Read the model definition and answer for the solid it produces. Units are mm, in the model's axes. A direction names the side the tool comes from. Give positions to 0.01 mm unless a question says otherwise; leave off trailing zeros. Loops run counter-clockwise (first coordinate to the right, second up) from the corner with the lowest first, then second, coordinate; pieces in that order, holes last. Notation, with made-up numbers: (7.25, 51) - (56.25, 51) arc R25 cw to (56.25, 72) - close; hole circle Ø4 at (3.25, -6.5). An arc over 180 degrees is marked (long way). Use a Markdown table: item, result. Add a question column.
Item 1: Which of the six approach directions +Z, -Z, +X, -X, +Y, -Y give full straight-line access (tool end or side, diameter ignored) to faces 4 (the face through (-12.97, -1.89, -1.45)), 5 (the face through (0.13, 4.08, 1.88)), 6 (the face through (13.07, -1.89, -1.45))?
Item 2: A cutting plane is placed at B-B (x = 2). Determine the outline of the cut face in (y, z) (3 decimals).
Item 3: A cutting plane is placed at C-C (z = 0). Determine the outline of the cut face in (x, y) (3 decimals), plus the area to 3 significant figures.
Item 4: Consider probe 1 along Z at (x, y) = (5.75, 0) (3 decimals); probe 2 along Z at (x, y) = (-8.5, 4.5); probe 3 along Y at (x, z) = (-8, -5). Determine where each line is inside the solid, lowest interval first. Write a range as [from, to].
Item 5: For a pull along Z with two mould halves and no side action, classify faces 1 (the face through (0.112, -2.808, -12.646)), 2 (the face through (16.51, 0, 0)), 3 (the face through (0.13, -3.67, -5.03)) as +Z half, -Z half, draft (parallel to the pull), parting line (faces both ways), or undercut.
Item 6: A cutting plane is placed at D-D (z = -3.81). Give the number of separate pieces and of enclosed holes in the cut face, plus the area to 3 significant figures.
Item 7: Each of these flat-tipped pins is pushed along its axis until it touches: P1, Ø4, axis at y = 6.6, z = 3.81, coming from the -X side; P2, Ø4, axis at x = -3, z = 10.5, coming from the -Y side; P3, Ø8.5, axis at y = -6.6, z = -3.81, coming from the -X side (3 decimals); P4, Ø5, axis at x = 5, z = -8.5, coming from the -Y side. Where does it stop, or does it pass through?
Item 8: A cutting plane is placed at A-A (y = 0). Determine the outline of the cut face in (x, z) (3 decimals), plus the area to 4 significant figures.
from build123d import *

# Parameters (mm, degrees)
F0_R     = 12.954
F0_R_2   = 2.38125
F1_DEPTH = 9.525
F2_DEPTH = 16.51
F3_R     = 3.175
F4_DEPTH = 26.036
F5_SIZE  = 1.524


with BuildPart() as f1:
    # F0 (on Right) → F1 (new body, symmetric)
    with BuildSketch(Plane.YZ):
        Circle(F0_R)
        Circle(F0_R_2, mode=Mode.SUBTRACT)
    extrude(amount=F1_DEPTH, both=True)

    # F0 (on Right) → F2 (join, symmetric)
    with BuildSketch(Plane.YZ):
        Circle(F0_R_2)
    extrude(amount=F2_DEPTH, both=True)

    # F3 (on face) → F4 (cut, through all)
    with BuildSketch(Plane.YZ.offset(9.525)):
        with Locations((0, 7.62)):
            Circle(F3_R)
        with Locations((-6.5991135768, 3.81)):
            Circle(F3_R)
        with Locations((-6.5991135768, -3.81)):
            Circle(F3_R)
        with Locations((0, -7.62)):
            Circle(F3_R)
        with Locations((6.5991135768, -3.81)):
            Circle(F3_R)
        with Locations((6.5991135768, 3.81)):
            Circle(F3_R)
    extrude(amount=-F4_DEPTH, mode=Mode.SUBTRACT)

    # F5
    f5_edges = [f1.edges().sort_by_distance(p)[0] for p in [
        (9.525, -12.954, 0),
        (-9.525, -12.954, 0),
    ]]
    chamfer(f5_edges, length=F5_SIZE)


solid = f1.part
Geometry says:
| question | item | result |
|---|---|---|
| 1 | face 4 | -X |
| 1 | face 5 | +X, -X |
| 1 | face 6 | +X |
| 2 | outline | circle Ø25.908 at (0, 0); hole circle Ø6.35 at (-6.599, -3.81); hole circle Ø6.35 at (-6.599, 3.81); hole circle Ø6.35 at (0, -7.62); hole circle Ø6.35 at (0, 7.62); hole circle Ø6.35 at (6.599, -3.81); hole circle Ø6.35 at (6.599, 3.81) |
| 3 | outline | (-16.51, -2.381) - (-9.525, -2.381) - (-9.525, -11.43) - (-8.001, -12.954) - (8.001, -12.954) - (9.525, -11.43) - (9.525, -2.381) - (16.51, -2.381) - (16.51, 2.381) - (9.525, 2.381) - (9.525, 11.43) - (8.001, 12.954) - (-8.001, 12.954) - (-9.525, 11.43) - (-9.525, 2.381) - (-16.51, 2.381) - close |
| 3 | area | 555 mm² |
| 4 | probe 1 | [-12.954, -10.795], [-4.445, 4.445], [10.795, 12.954] |
| 4 | probe 2 | [-11.61, -6.19], [-1.43, 1.43], [6.19, 11.61] |
| 4 | probe 3 | [-11.95, -9.54], [-3.66, -1.79], [1.79, 3.66], [9.54, 11.95] |
| 5 | face 1 | parting line |
| 5 | face 2 | draft |
| 5 | face 3 | undercut |
| 6 | separate pieces | 3 |
| 6 | enclosed holes | 0 |
| 6 | area | 225 mm² |
| 7 | P1 | through |
| 7 | P2 | y = -9.78 |
| 7 | P3 | x = -9.525 |
| 7 | P4 | y = -11.48 |
| 8 | outline | (-16.51, -2.381) - (-9.525, -2.381) - (-9.525, -4.445) - (9.525, -4.445) - (9.525, -2.381) - (16.51, -2.381) - (16.51, 2.381) - (9.525, 2.381) - (9.525, 4.445) - (-9.525, 4.445) - (-9.525, 2.381) - (-16.51, 2.381) - close; (-9.525, -11.43) - (-8.001, -12.954) - (8.001, -12.954) - (9.525, -11.43) - (9.525, -10.795) - (-9.525, -10.795) - close; (-9.525, 10.795) - (9.525, 10.795) - (9.525, 11.43) - (8.001, 12.954) - (-8.001, 12.954) - (-9.525, 11.43) - close |
| 8 | area | 313.5 mm² |
